```python
from build123d import *

# Parameters (mm, degrees)
F0_W      = 50
F0_H      = 50
F1_DEPTH  = 50
F2_R      = 22.5
F3_DEPTH  = 5
F4_R      = 17.5
F5_DEPTH  = 5
F6_R      = 12.5
F7_DEPTH  = 5
F8_R      = 22.5
F9_DEPTH  = 5
F10_R     = 17.5
F11_DEPTH = 5
F12_R     = 12.5
F13_DEPTH = 5
F14_R     = 22.5
F15_DEPTH = 5
F16_R     = 17.5
F17_DEPTH = 5
F18_R     = 12.5
F19_DEPTH = 5
F20_R     = 22.5
F21_DEPTH = 5
F22_R     = 17.5
F23_DEPTH = 5
F24_R     = 12.5
F25_DEPTH = 5
F26_R     = 22.5
F27_DEPTH = 5
F28_R     = 17.5
F29_DEPTH = 5
F30_R     = 12.5
F31_DEPTH = 5
F32_R     = 22.5
F33_DEPTH = 5
F34_R     = 17.5
F35_DEPTH = 5
F36_R     = 12.5
F37_DEPTH = 5


with BuildPart() as f1:
    # F0 (on Top) → F1 (new body)
    with BuildSketch(Plane.XY):
        with Locations((25, 25)):
            Rectangle(F0_W, F0_H)
    extrude(amount=F1_DEPTH)

    # F2 (on face) → F3 (cut)
    with BuildSketch(Plane.XY.offset(50)):
        with Locations((25, 25)):
            Circle(F2_R)
    extrude(amount=-F3_DEPTH, mode=Mode.SUBTRACT)

    # F4 (on face) → F5 (cut)
    with BuildSketch(Plane.XY.offset(45)):
        with Locations((25, 25)):
            Circle(F4_R)
    extrude(amount=-F5_DEPTH, mode=Mode.SUBTRACT)

    # F6 (on face) → F7 (cut)
    with BuildSketch(Plane.XY.offset(40)):
        with Locations((25, 25)):
            Circle(F6_R)
    extrude(amount=-F7_DEPTH, mode=Mode.SUBTRACT)

    # F8 (on face) → F9 (cut)
    with BuildSketch(Plane(origin=(0, 0, 0), x_dir=(0, -1, 0), z_dir=(-1, 0, 0))):
        with Locations((-25, 25)):
            Circle(F8_R)
    extrude(amount=-F9_DEPTH, mode=Mode.SUBTRACT)

    # F10 (on face) → F11 (cut)
    with BuildSketch(Plane(origin=(5, 0, 0), x_dir=(0, -1, 0), z_dir=(-1, 0, 0))):
        with Locations((-25, 25)):
            Circle(F10_R)
    extrude(amount=-F11_DEPTH, mode=Mode.SUBTRACT)

    # F12 (on face) → F13 (cut)
    with BuildSketch(Plane(origin=(10, 0, 0), x_dir=(0, -1, 0), z_dir=(-1, 0, 0))):
        with Locations((-25, 25)):
            Circle(F12_R)
    extrude(amount=-F13_DEPTH, mode=Mode.SUBTRACT)

    # F14 (on face) → F15 (cut)
    with BuildSketch(Plane.XZ):
        with Locations((25, 25)):
            Circle(F14_R)
    extrude(amount=-F15_DEPTH, mode=Mode.SUBTRACT)

    # F16 (on face) → F17 (cut)
    with BuildSketch(Plane.XZ.offset(-5)):
        with Locations((25, 25)):
            Circle(F16_R)
    extrude(amount=-F17_DEPTH, mode=Mode.SUBTRACT)

    # F18 (on face) → F19 (cut)
    with BuildSketch(Plane.XZ.offset(-10)):
        with Locations((25, 25)):
            Circle(F18_R)
    extrude(amount=-F19_DEPTH, mode=Mode.SUBTRACT)

    # F20 (on face) → F21 (cut)
    with BuildSketch(Plane.YZ.offset(50)):
        with Locations((25, 25)):
            Circle(F20_R)
    extrude(amount=-F21_DEPTH, mode=Mode.SUBTRACT)

    # F22 (on face) → F23 (cut)
    with BuildSketch(Plane.YZ.offset(45)):
        with Locations((25, 25)):
            Circle(F22_R)
    extrude(amount=-F23_DEPTH, mode=Mode.SUBTRACT)

    # F24 (on face) → F25 (cut)
    with BuildSketch(Plane.YZ.offset(40)):
        with Locations((25, 25)):
            Circle(F24_R)
    extrude(amount=-F25_DEPTH, mode=Mode.SUBTRACT)

    # F26 (on face) → F27 (cut)
    with BuildSketch(Plane(origin=(0, 50, 0), x_dir=(-1, 0, 0), z_dir=(0, 1, 0))):
        with Locations((-25, 25)):
            Circle(F26_R)
    extrude(amount=-F27_DEPTH, mode=Mode.SUBTRACT)

    # F28 (on face) → F29 (cut)
    with BuildSketch(Plane(origin=(0, 45, 0), x_dir=(-1, 0, 0), z_dir=(0, 1, 0))):
        with Locations((-25, 25)):
            Circle(F28_R)
    extrude(amount=-F29_DEPTH, mode=Mode.SUBTRACT)

    # F30 (on face) → F31 (cut)
    with BuildSketch(Plane(origin=(0, 40, 0), x_dir=(-1, 0, 0), z_dir=(0, 1, 0))):
        with Locations((-25, 25)):
            Circle(F30_R)
    extrude(amount=-F31_DEPTH, mode=Mode.SUBTRACT)

    # F32 (on face) → F33 (cut)
    with BuildSketch(Plane(origin=(0, 0, 0), x_dir=(1, 0, 0), z_dir=(0, 0, -1))):
        with Locations((25, -25)):
            Circle(F32_R)
    extrude(amount=-F33_DEPTH, mode=Mode.SUBTRACT)

    # F34 (on face) → F35 (cut)
    with BuildSketch(Plane(origin=(0, 0, 5), x_dir=(1, 0, 0), z_dir=(0, 0, -1))):
        with Locations((25, -25)):
            Circle(F34_R)
    extrude(amount=-F35_DEPTH, mode=Mode.SUBTRACT)

    # F36 (on face) → F37 (cut)
    with BuildSketch(Plane(origin=(0, 0, 10), x_dir=(1, 0, 0), z_dir=(0, 0, -1))):
        with Locations((25, -25)):
            Circle(F36_R)
    extrude(amount=-F37_DEPTH, mode=Mode.SUBTRACT)


solid = f1.part
```
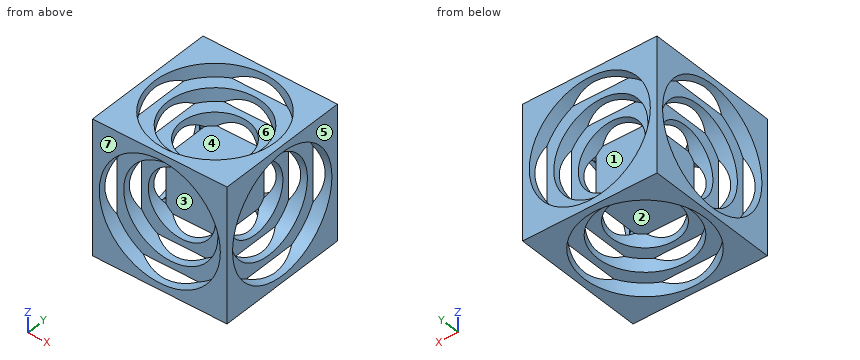
Source: CAD feature listing. Evaluate the final solid. Frame: model axes, mm. Face numbers are marked on the shaded views. A direction names the side the tool comes from. Round coordinates to 2 decimals unless told otherwise and drop trailing zeros. Loops run counter-clockwise (first coordinate to the right, second up) from the corner with the lowest first, then second, coordinate; pieces in that order, holes last.
(1) Section query C-C (x = 46.5). Output: boundary loops of the cut face in (y, z).
From the geometry:
outline: (0, 0) - (18.37, 0) - (18.37, 3.5) arc R22.5 cw to (3.5, 18.37) - (0, 18.37) - close; (0, 31.63) - (3.5, 31.63) arc R22.5 cw to (18.37, 46.5) - (18.37, 50) - (0, 50) - close; (31.63, 0) - (50, 0) - (50, 18.37) - (46.5, 18.37) arc R22.5 cw to (31.63, 3.5) - close; (31.63, 46.5) arc R22.5 cw to (46.5, 31.63) - (50, 31.63) - (50, 50) - (31.63, 50) - close
(2) Contact query for flat-ended pins moving along their axis: pin 1 Ø22.5 at (y, z) = (25, 25) entering from -X; pin 2 Ø22 at (x, y) = (22.5, 23) entering from -Z; pin 3 Ø2 at (y, z) = (39.5, 20) entering from +X. Output: stop coordinate, or through.
From the geometry:
pin 1: stops at x = 15
pin 2: stops at z = 10
pin 3: stops at x = 40
(3) Material intervals for probe 1 along X at (y, z) = (12.05, 25); probe 2 along Z at (x, y) = (34, 20); probe 3 along Y at (x, z) = (25, 2), sorted ascending.
From the geometry:
probe 1: x = 10 to 12.5, 37.5 to 40
probe 2: z = 15 to 35
probe 3: y = 0 to 2.5, 47.5 to 50
(4) Access query for the marked faces 1, 2, 3 and 4. Directions: +Z, -Z, +X, -X, +Y, -Y. A direction counts if a zero-diameter tool reaches every point of the face in a straight line with its end or side. Return the directions, or none.
From the geometry:
face 1: +Y
face 2: -Z
face 3: -Y
face 4: +Z
(5) Section query A-A (x = 25). Give the number of separate pieces and of enclosed holes in the cut face, and give its area (3 significant figures).
From the geometry:
separate pieces: 13
enclosed holes: 0
area: 475 mm2
(6) Pull-direction query (X, two-part tool) for the marked faces 5, 6 and 7; classes: +X half, -X half, draft (parallel to the pull), parting line (faces both ways), or undercut.
From the geometry:
face 5: +X half
face 6: undercut
face 7: draft
